Autodesk Inventor part; units mm, degrees
ref_plane "YZ Plane" through (0, 0, 0) normal (1, 0, 0) x (0, 1, 0)
ref_plane "XZ Plane" through (0, 0, 0) normal (0, 1, 0) x (-1, 0, 0)
ref_plane "XY Plane" through (0, 0, 0) normal (0, 0, 1) x (1, 0, 0)
sketch "Sketch1" plane through (0, 0, 0) normal (0, 0, 1) x (1, 0, 0)
  circle A0 centre (58.7079, -22.221) radius 2.1844
  circle A1 centre (67.9751, -13.5372) radius 2.1844
  circle A2 centre (4.1043, 3.1638) radius 2.1844
  circle A3 centre (4.1043, -9.5362) radius 2.1844
  circle A4 centre (15.8718, 42.0658) radius 2.1844
  circle A5 centre (6.6046, 33.3819) radius 2.1844
  arc A6 (2.2627, 38.0155) -> (0.2654, 33.7512) centre (6.6046, 33.3819) ccw
  arc A7 (20.5054, 46.4077) -> (11.5299, 46.6994) centre (15.8718, 42.0658) ccw
  arc A8 (-2.235, -9.1669) -> (2.6674, -15.7215) centre (4.1043, -9.5362) ccw
  arc A9 (57.2711, -28.4063) -> (63.0499, -26.8546) centre (58.7079, -22.221) ccw
  arc A10 (72.317, -18.1707) -> (72.6087, -9.1952) centre (67.9751, -13.5372) ccw
  line L0 (20.5054, 46.4077) -> (72.6087, -9.1952)
  line L1 (72.317, -18.1707) -> (63.0499, -26.8546)
  line L2 (2.6674, -15.7215) -> (57.2711, -28.4063)
  line L3 (0.2654, 33.7512) -> (-2.235, -9.1669)
  line L4 (2.2627, 38.0155) -> (11.5299, 46.6994)
  circle A11 centre (32.9479, 14.556) radius 2.1844
  dimension "d8" = 12.7
  dimension "d9" = 12.7
  dimension "d10" = 12.7
  dimension "d11" = 12.7
  dimension "d12" = 12.7
  dimension "d14" = 4.3688
extrude "Extrusion1" add sketch "Sketch1" along normal blind 1.5875
properties part number "2-Gearbox"
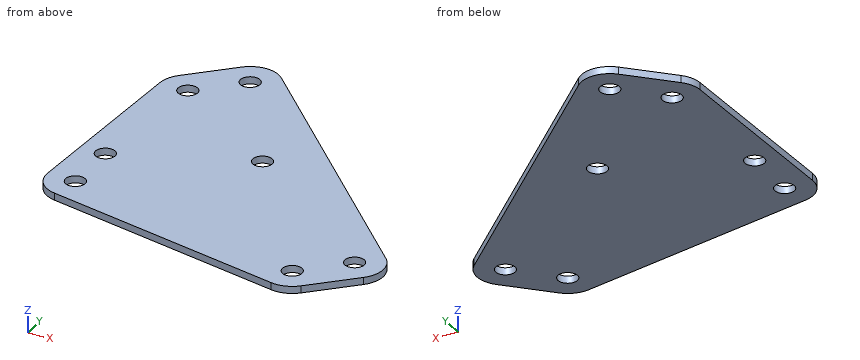
Geometry check sheet. Reference: the model listing, model coordinates, mm. Coordinates: 2 decimals unless noted, no trailing zeros. Loops run counter-clockwise (first coordinate to the right, second up) from the corner with the lowest first, then second, coordinate; pieces in that order, holes last. Notation, with made-up numbers: (72.5, 21) - (125.5, 21) arc R23 ccw to (125.5, 43) - close; hole circle Ø5 at (39, -12.75). An arc over 180 degrees is marked (long way). Use one line per item in the form item = value. Start each with the question number.
Item 1: Section check C-C, the plane y = 2. Enter the section's corners in (x, z).
Item 2: Section check B-B, the plane x = 68.5. Enter the section's corners in (y, z).
Item 3: Section check D-D, the plane y = 24. Enter the section's corners in (x, z).
Item 4: Section check A-A, the plane z = 0.45. Enter the section's corners in (x, y) (1 decimal), and give its area (3 significant figures).
Item 5: Thickness scan on probe 1 along Y at (x, z) = (59, 1.3); probe 2 along Y at (x, z) = (3.5, 0.2); probe 3 along Y at (x, z) = (31.5, 0.3). Record the ranges inside material, lowest first.
Computed:
q1.outline = (-1.58, 0) - (2.26, 0) - (2.26, 1.59) - (-1.58, 1.59) - close; (5.95, 0) - (62.12, 0) - (62.12, 1.59) - (5.95, 1.59) - close
q2.outline = (-21.75, 0) - (-15.66, 0) - (-15.66, 1.59) - (-21.75, 1.59) - close; (-11.42, 0) - (-4.81, 0) - (-4.81, 1.59) - (-11.42, 1.59) - close
q3.outline = (-0.3, 0) - (41.5, 0) - (41.5, 1.59) - (-0.3, 1.59) - close
q4.outline = (-2.2, -9.2) arc R6.3 ccw to (2.7, -15.7) - (57.3, -28.4) arc R6.4 ccw to (63, -26.9) - (72.3, -18.2) arc R6.4 ccw to (72.6, -9.2) - (20.5, 46.4) arc R6.3 ccw to (11.5, 46.7) - (2.3, 38) arc R6.3 ccw to (0.3, 33.8) - close; hole circle Ø4.4 at (4.1, -9.5); hole circle Ø4.4 at (4.1, 3.2); hole circle Ø4.4 at (6.6, 33.4); hole circle Ø4.4 at (15.9, 42.1); hole circle Ø4.4 at (32.9, 14.6); hole circle Ø4.4 at (58.7, -22.2); hole circle Ø4.4 at (68, -13.5)
q4.area = 3,450 mm2
q5.probe_1 = -28.56 to -24.39, -20.06 to 5.33
q5.probe_2 = -15.91 to -11.64, -7.44 to 1.06, 5.26 to 39.17
q5.probe_3 = -22.42 to 12.92, 16.19 to 34.67
